Geometry check sheet. Reference: drawing and pictorial views, mm from the part's lowest x, y, z. Give positions to 0.01 mm unless a question says otherwise; leave off trailing zeros. Write each loop counter-clockwise with the first axis right and the second up, starting at its lowest first coordinate (ties: lowest second). Pieces come first, ordered by that corner, then holes. Notation, with made-up numbers: (65.5, 56) -> (104.5, 56) arc R21 ccw to (104.5, 60) -> close; hole circle Ø9 at (88, 74.5). An arc over 180 degrees is marked (long way). Use a Markdown table: item, result. Add a question column.
1. Cross-section at A-A (z = 8). Enter the section's corners in (x, y), then the cut area to 3 significant figures.
2. Cross-section at B-B (x = 8). Enter the section's corners in (y, z), then the cut area to 3 significant figures.
3. Scan lines: probe 1 along X at (y, z) = (0.3, 8); probe 2 along Z at (x, y) = (8, 0.35); probe 3 along X at (y, z) = (0.45, 10.75). Record each from-to range of solid material in increasing order. Write a range as [from, to].
4. Cross-section at C-C (z = 3.75). Enter the section's corners in (x, y), then the cut area to 3 significant figures.
5. Cross-section at D-D (y = 0.4). Enter the section's corners in (x, z), then the cut area to 3 significant figures.
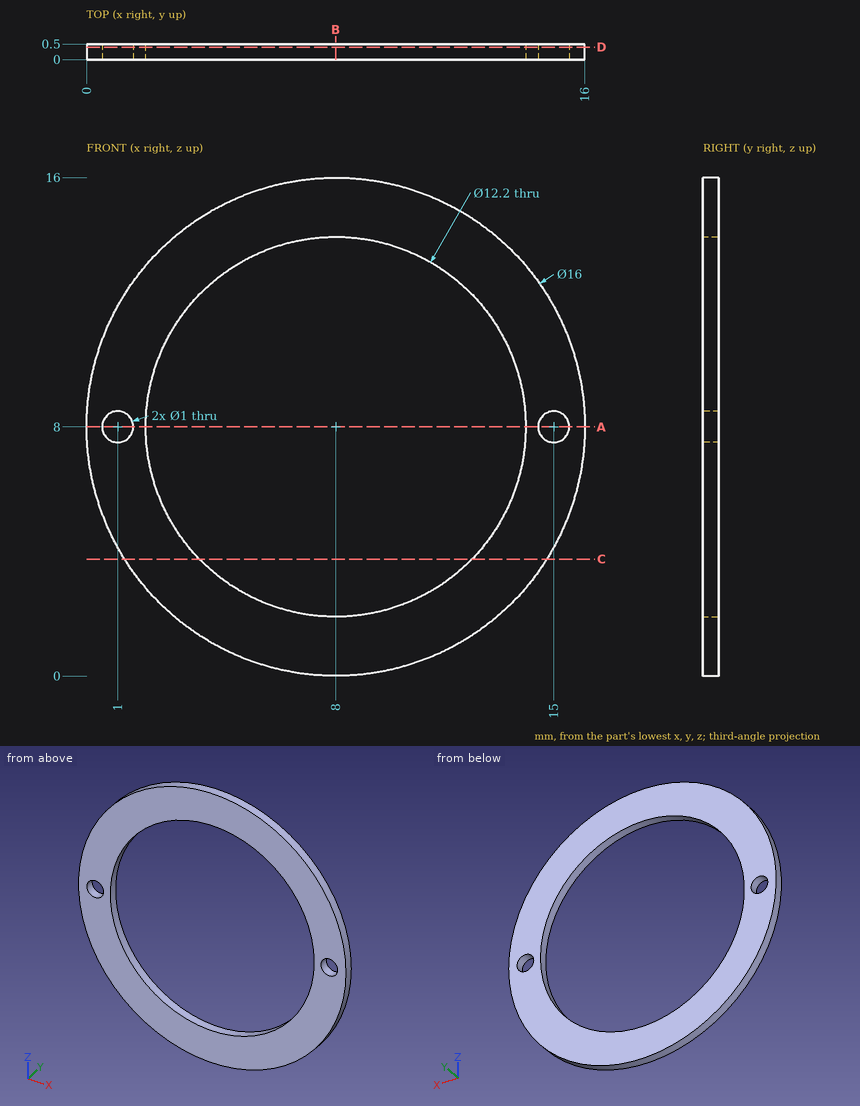
Worked answers:
| question | item | result |
|---|---|---|
| 1 | outline | (0, 0) -> (0.5, 0) -> (0.5, 0.5) -> (0, 0.5) -> close; (1.5, 0) -> (1.9, 0) -> (1.9, 0.5) -> (1.5, 0.5) -> close; (14.1, 0) -> (14.5, 0) -> (14.5, 0.5) -> (14.1, 0.5) -> close; (15.5, 0) -> (16, 0) -> (16, 0.5) -> (15.5, 0.5) -> close |
| 1 | area | 0.900 mm² |
| 2 | outline | (0, 0) -> (0.5, 0) -> (0.5, 1.9) -> (0, 1.9) -> close; (0, 14.1) -> (0.5, 14.1) -> (0.5, 16) -> (0, 16) -> close |
| 2 | area | 1.90 mm² |
| 3 | probe 1 | x = [0, 0.5], [1.5, 1.9], [14.1, 14.5], [15.5, 16] |
| 3 | probe 2 | z = [0, 1.9], [14.1, 16] |
| 3 | probe 3 | x = [0.49, 2.56], [13.44, 15.51] |
| 4 | outline | (1.22, 0) -> (3.62, 0) -> (3.62, 0.5) -> (1.22, 0.5) -> close; (12.38, 0) -> (14.78, 0) -> (14.78, 0.5) -> (12.38, 0.5) -> close |
| 4 | area | 2.40 mm² |
| 5 | outline | circle Ø16 at (8, 8); hole circle Ø1 at (1, 8); hole circle Ø12.2 at (8, 8); hole circle Ø1 at (15, 8) |
| 5 | area | 82.6 mm² |
